from build123d import *

# Parameters (mm, degrees)
SKETCH2_R           = 4.4704
SKETCH2_R_2         = 1.905
BOSS_EXTRUDE1_DEPTH = 1.397
SKETCH3_R           = 3.052127004
SKETCH3_R_2         = 1.905
BOSS_EXTRUDE2_DEPTH = 4.826


with BuildPart() as part:
    # Sketch2 → Boss-Extrude1 (new body)
    # profile 1 of 3: a face of its own
    with BuildSketch(Plane.XY):
        Circle(SKETCH2_R)
        Circle(SKETCH2_R_2, mode=Mode.SUBTRACT)
    # profile 2 of 3: a face of its own
    with BuildSketch(Plane.XY):
        with BuildLine():
            ThreePointArc((-4.185765955, 1.569662233), (0, 4.4704), (4.185765955, 1.569662233))
            ThreePointArc((4.185765955, 1.569662233), (3.606794054, 4.7625), (4.185765955, 7.955337767))
            ThreePointArc((4.185765955, 7.955337767), (0, 5.0546), (-4.185765955, 7.955337767))
            ThreePointArc((-4.185765955, 7.955337767), (-3.606794054, 4.7625), (-4.185765955, 1.569662233))
        make_face()
    # profile 3 of 3: a face of its own
    with BuildSketch(Plane.XY):
        with Locations((0, 9.525)):
            Circle(SKETCH2_R)
        with Locations((0, 9.525)):
            Circle(SKETCH2_R_2, mode=Mode.SUBTRACT)
    boss_extrude1 = extrude(amount=BOSS_EXTRUDE1_DEPTH)

    # Sketch3 → Boss-Extrude2 (add)
    with BuildSketch(Plane.XY.offset(1.397)):
        Circle(SKETCH3_R)
        Circle(SKETCH3_R_2, mode=Mode.SUBTRACT)
    extrude(amount=BOSS_EXTRUDE2_DEPTH)

    # Mirror1: Boss-Extrude1 across plane
    add(boss_extrude1.mirror(Plane.XY.offset(3.81)))


solid = part.part
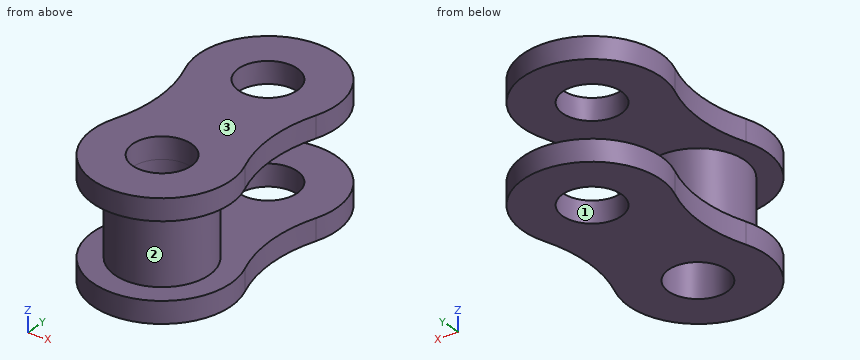
Input: part model. Units: mm. Frame: model coordinates. Face numbers are marked on the shaded views. Give positions to 0.01 mm unless a question says otherwise; leave off trailing zeros. Order: outer loops, then holes, each group sorted by start corner. A loop starts at its lowest first (then second) coordinate and runs counter-clockwise, first axis right, second up. Notation, with made-up numbers: (-39, 70.25) - (8, 70.25) arc R18 cw to (8, 94.25) - close; hole circle Ø7 at (-1.5, 15). An arc over 180 degrees is marked (long way). Write each question's results on one line, items separated by ' | '.
Item 1: Section D-D (x = 2.75). Return loops of the section in (y, z).
A:
outline: (-3.52, 0) - (13.05, 0) - (13.05, 1.4) - (1.32, 1.4) - (1.32, 6.22) - (13.05, 6.22) - (13.05, 7.62) - (-3.52, 7.62) - (-3.52, 6.22) - (-1.32, 6.22) - (-1.32, 1.4) - (-3.52, 1.4) - close
Item 2: Contact query for flat-ended pins moving along their axis: pin 1 Ø4 at (x, z) = (2.5, 1) entering from -Y; pin 2 Ø3 at (x, z) = (-1, 4) entering from -Y. Output: stop coordinate, or through.
A:
pin 1: stops at y = -4.44 | pin 2: stops at y = -3.05
Item 3: Section C-C (z = 5.75). Return loops of the section in (x, y) (3 decimals).
A:
outline: circle Ø6.104 at (0, 0); hole circle Ø3.81 at (0, 0)
Item 4: Material intervals for line 1 along Y through (x, z) = (0, 6.8) (3 decimals); line 2 along Z through (x, y) = (-0.75, 3.75); line 3 along Y through (x, z) = (0, 3.75) (3 decimals), sorted ascending.
A:
line 1: y = -4.47 to -1.905, 1.905 to 7.62, 11.43 to 13.995 | line 2: z = 0 to 1.4, 6.22 to 7.62 | line 3: y = -3.052 to -1.905, 1.905 to 3.052
Item 5: Section A-A (y = 0). Return loops of the section in (x, z) (3 decimals).
A:
outline: (-4.47, 0) - (-1.905, 0) - (-1.905, 7.62) - (-4.47, 7.62) - (-4.47, 6.223) - (-3.052, 6.223) - (-3.052, 1.397) - (-4.47, 1.397) - close; (1.905, 0) - (4.47, 0) - (4.47, 1.397) - (3.052, 1.397) - (3.052, 6.223) - (4.47, 6.223) - (4.47, 7.62) - (1.905, 7.62) - close
Item 6: Draft query along Y for the marked faces 1, 2 and 3. Return one class per face: released by +Y, released by -Y, zero draft, split by the parting line, or undercut.
A:
face 1: undercut | face 2: split by the parting line | face 3: zero draft
Item 7: Section B-B (x = 0). Return loops of the section in (y, z) (3 decimals), and give its area (3 significant figures).
A:
outline: (-4.47, 0) - (-1.905, 0) - (-1.905, 7.62) - (-4.47, 7.62) - (-4.47, 6.223) - (-3.052, 6.223) - (-3.052, 1.397) - (-4.47, 1.397) - close; (1.905, 0) - (7.62, 0) - (7.62, 1.397) - (3.052, 1.397) - (3.052, 6.223) - (7.62, 6.223) - (7.62, 7.62) - (1.905, 7.62) - close; (11.43, 0) - (13.995, 0) - (13.995, 1.397) - (11.43, 1.397) - close; (11.43, 6.223) - (13.995, 6.223) - (13.995, 7.62) - (11.43, 7.62) - close | area: 41.4 mm^2
